Here's the drawing with two shaded views (mm, measured from the low corner). I have some questions. A direction names the side the tool comes from. Coordinates: 2 decimals unless noted, no trailing zeros. Write each loop counter-clockwise with the first axis right and the second up, starting at its lowest first coordinate (ties: lowest second). Pieces come first, ordered by that corner, then holes. Notation, with made-up numbers: (2, -6) - (60, -6) arc R18 cw to (60, 27) - close; hole circle Ø7 at (-27, 31.25). An arc over 180 degrees is marked (long way). Answer in a Markdown table with one row per item. Add a question column.
Item 1: We'd pull the mould along X, two halves only. Please class the marked faces 4, 5 and 6: +X half, -X half, draft (parallel to the pull), parting line (faces both ways), or undercut.
Item 2: I'm going to push flat-ended pins straight in: pin 1 (6 mm diameter, centred on y = 20, z = 25.5, fed in from +X); pin 2 (3 mm diameter, centred on y = 29, z = 27.5, fed in from -X); pin 3 (5 mm diameter, centred on x = 12, z = 11.5, fed in from -Y) (1 decimal). Where does each tip first touch, or does it pass through?
Item 3: Imagine slicing it at B-B (z = 11). Please give me the cut outline in (x, y).
Item 4: Which directions (+Z, -Z, +X, -X, +Y, -Y) give clear straight access to the entire face, cutting with the end or side of a thin tool? Please do the marked faces 1, 2 and 3.
Item 5: Imagine slicing it at A-A (z = 27.5). Please give me the cut outline in (x, y).
Item 6: If I drill on probe 1 along Y at (x, z) = (29, 20); probe 2 along X at (y, z) = (24.5, 16.5); probe 3 along Y at (x, z) = (35.5, 18) (1 decimal), over which ranges is the centre line in solid material (lowest first)? Write a range as from..to.
Item 7: Imagine slicing it at C-C (z = 18.5). Please give me the cut outline in (x, y), plus the area to 3 significant figures.
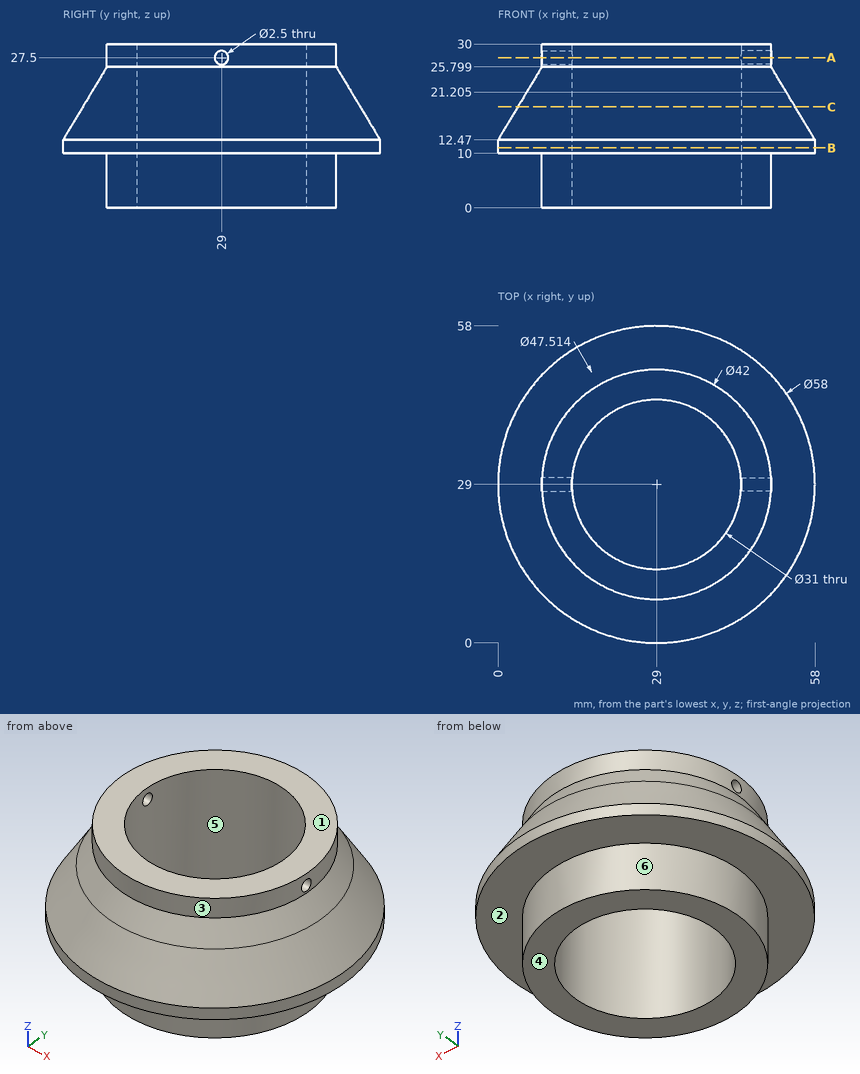
Here are the results:
| question | item | result |
|---|---|---|
| 1 | face 4 | draft |
| 1 | face 5 | undercut |
| 1 | face 6 | parting line |
| 2 | pin 1 | stops at x = 50.47 |
| 2 | pin 2 | stops at x = 8 |
| 2 | pin 3 | stops at y = 3.9 |
| 3 | outline | circle Ø58 at (29, 29); hole circle Ø31 at (29, 29) |
| 4 | face 1 | +Z, +X, -X, +Y, -Y |
| 4 | face 2 | -Z |
| 4 | face 3 | +Z |
| 5 | outline | (8.04, 27.75) arc R21 ccw to (49.96, 27.75) - (44.45, 27.75) arc R15.5 cw to (13.55, 27.75) - close; (8.04, 30.25) - (13.55, 30.25) arc R15.5 cw to (44.45, 30.25) - (49.96, 30.25) arc R21 ccw to start |
| 6 | probe 1 | y = 4.52..13.5, 44.5..53.48 |
| 6 | probe 2 | x = 2.8..14.17, 43.83..55.2 |
| 6 | probe 3 | y = 4.2..14.9, 43.1..53.8 |
| 7 | outline | circle Ø50.76 at (29, 29); hole circle Ø31 at (29, 29) |
| 7 | area | 1,270 mm2 |
